Autodesk Inventor part; units mm, degrees
ref_plane "YZ Plane" through (0, 0, 0) normal (1, 0, 0) x (0, 1, 0)
ref_plane "XZ Plane" through (0, 0, 0) normal (0, 1, 0) x (-1, 0, 0)
ref_plane "XY Plane" through (0, 0, 0) normal (0, 0, 1) x (1, 0, 0)
sketch "Sketch1" plane through (0, 0, 0) normal (0, 0, 1) x (1, 0, 0)
  line L0 (-3.43, -6.35) -> (3.43, -6.35)
  line L1 (3.43, -6.35) -> (3.43, 6.35)
  line L2 (3.43, 6.35) -> (-3.43, 6.35)
  line L3 (-3.43, 6.35) -> (-3.43, -6.35)
  line L4 (-3.43, -6.35) -> (3.43, 6.35) construction
  line L5 (3.43, -6.35) -> (-3.43, 6.35) construction
  point P0 (0, 0)
  dimension "d0" = 6.86
  dimension "d1" = 12.7
extrude "Extrusion1" add sketch "Sketch1" against normal blind 8.89
sketch "Sketch2" plane through (0, 0, 0) normal (0, 0, 1) x (1, 0, 0)
  circle A0 centre (0, 0) radius 3.175
  dimension "d35" = 6.35
extrude "Extrusion2" add sketch "Sketch2" along normal blind 8.89
sketch "Sketch3" plane through (0, 0, -8.89) normal (0, 0, -1) x (-1, 0, 0)
  line L0 (-1.015, -0.38) -> (1.015, -0.38)
  line L1 (1.015, -0.38) -> (1.015, 0.38)
  line L2 (1.015, 0.38) -> (-1.015, 0.38)
  line L3 (-1.015, 0.38) -> (-1.015, -0.38)
  line L4 (-1.015, -0.38) -> (1.015, 0.38) construction
  line L5 (1.015, -0.38) -> (-1.015, 0.38) construction
  line L6 (-1.015, -5.08) -> (1.015, -5.08)
  line L7 (1.015, -5.08) -> (1.015, -4.32)
  line L8 (1.015, -4.32) -> (-1.015, -4.32)
  line L9 (-1.015, -4.32) -> (-1.015, -5.08)
  line L10 (-1.015, -5.08) -> (1.015, -4.32) construction
  line L11 (1.015, -5.08) -> (-1.015, -4.32) construction
  line L12 (-1.015, -9.78) -> (1.015, -9.78) construction
  line L13 (1.015, -9.78) -> (1.015, -9.02) construction
  line L14 (1.015, -9.02) -> (-1.015, -9.02) construction
  line L15 (-1.015, -9.02) -> (-1.015, -9.78) construction
  line L16 (-1.015, -9.78) -> (1.015, -9.02) construction
  line L17 (1.015, -9.78) -> (-1.015, -9.02) construction
  line L18 (-1.015, 4.32) -> (1.015, 4.32)
  line L19 (1.015, 4.32) -> (1.015, 5.08)
  line L20 (1.015, 5.08) -> (-1.015, 5.08)
  line L21 (-1.015, 5.08) -> (-1.015, 4.32)
  line L22 (-1.015, 4.32) -> (1.015, 5.08) construction
  line L23 (1.015, 4.32) -> (-1.015, 5.08) construction
  point P0 (0, 0)
  point P1 (0, 4.7)
  dimension "d6" = 2.03
  dimension "d7" = 0.76
  dimension "d10" = 4.7
  dimension "d17" = 4.7
extrude "Extrusion3" add sketch "Sketch3" along normal blind 3.96
sketch "Sketch4" plane through (-1.015, 5.08, -8.89) normal (0, 1, 0) x (1, 0, 0)
  line L0 (2.03, 0) -> (2.03, 3.96)
  line L1 (0, 3.96) -> (2.03, 3.96)
  circle A0 centre (1.015, 2.96) radius 0.5
  point P0 (1.015, -8.89)
  dimension "d24" = 1
  dimension "d25" = 1
  dimension "d26" = 1.015
extrude "Extrusion4" cut sketch "Sketch4" against normal through all
sketch "Sketch6" plane through (0, 0, 8.89) normal (0, 0, 1) x (1, 0, 0)
  circle A0 centre (0, 0) radius 1.46
  circle A1 centre (0, 0) radius 3.175
  dimension "d29" = 2.92
extrude "Extrusion5" add sketch "Sketch6" along normal blind 10.41 contours A0
fillet "Fillet1" radius 1.46 1 edges at (-1.46, 0, 19.3)
thread "Thread1"
sketch "Sketch7" plane through (-1.015, -5.08, -8.89) normal (0, -1, 0) x (1, 0, 0)
  circle A0 centre (1.015, -2.96) radius 0.5
sketch "Sketch8" plane through (-1.015, -0.38, -8.89) normal (0, -1, 0) x (1, 0, 0)
  circle A0 centre (1.015, -2.96) radius 0.5
sketch "Sketch9" plane through (-1.015, 4.32, -8.89) normal (0, -1, 0) x (1, 0, 0)
  circle A0 centre (1.015, -2.96) radius 0.5
properties part number "1MS2" material "Aluminum"
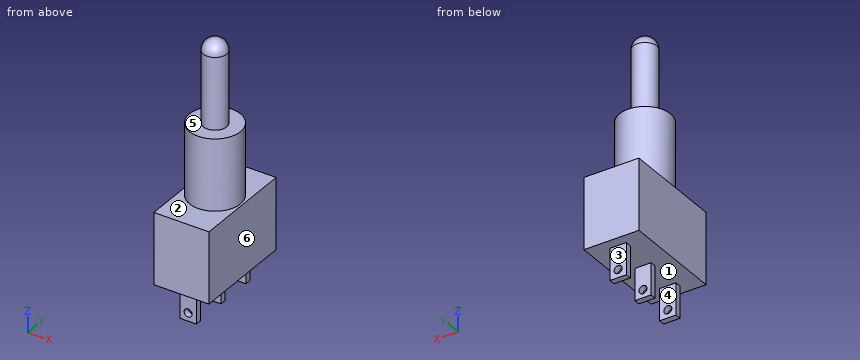
The listing builds one solid part. Answer for the finished solid, in the listing's coordinates (mm). Face numbers are marked on the shaded views. A direction names the side the tool comes from. Give positions to 0.01 mm unless a question says otherwise; leave off trailing zeros. Write each loop counter-clockwise with the first axis right and the second up, starting at its lowest first coordinate (ties: lowest second). Pieces come first, ordered by that corner, then holes. Notation, with made-up numbers: (-13.5, -2.75) - (40.5, -2.75) arc R13 cw to (40.5, 20.25) - close; hole circle Ø1 at (-28, 25.5). An arc over 180 degrees is marked (long way). Use a Markdown table: item, result.
1. A tool of negligible diameter and unlimited length cuts with its end or side. For the marked faces 4, 5 and 6, from which of +Z, -Z, +X, -X, +Y, -Y can it reach the whole face along a straight path? Write none if from no direction.
Values follow:
| item | result |
|---|---|
| face 4 | -Z, +X, -X |
| face 5 | +Z |
| face 6 | +Z, -Z, +X, +Y, -Y |
2. Each of these flat-tipped pins is pushed along its axis until it touches: P1, Ø2, axis at x = 0.5, z = -11, coming from the +Y side; P2, Ø2, axis at x = 0.5, z = -10, coming from the -Y side; P3, Ø0.8, axis at y = -4.5, z = -10.5, coming from the +X side (3 decimals). Where does it stop, or does it pass through?
Values follow:
| item | result |
|---|---|
| P1 | stops at y = 5.08 |
| P2 | stops at y = -5.08 |
| P3 | stops at x = 1.015 |
3. Section B-B on y = 0 is taken. Write down the section's boundary in (x, z) (3 decimals), plus the area to 3 significant figures.
Values follow:
| item | result |
|---|---|
| outline | (-3.43, -8.89) - (-1.015, -8.89) - (-1.015, -12.85) - (1.015, -12.85) - (1.015, -8.89) - (3.43, -8.89) - (3.43, 0) - (3.175, 0) - (3.175, 8.89) - (1.46, 8.89) - (1.46, 17.84) arc R1.46 ccw to (-1.46, 17.84) - (-1.46, 8.89) - (-3.175, 8.89) - (-3.175, 0) - (-3.43, 0) - close; hole circle Ø1 at (0, -11.85) |
| area | 154 mm² |
4. Section C-C on x = -2 is taken. Write down the section's boundary in (y, z), plus the area to 3 significant figures.
Values follow:
| item | result |
|---|---|
| outline | (-6.35, -8.89) - (6.35, -8.89) - (6.35, 0) - (2.47, 0) - (2.47, 8.89) - (-2.47, 8.89) - (-2.47, 0) - (-6.35, 0) - close |
| area | 157 mm² |
5. Section D-D on x = 0 is taken. Count the separate pieces of the cut face and the enclosed holes in it, plus the area to 3 significant figures.
Values follow:
| item | result |
|---|---|
| separate pieces | 4 |
| enclosed holes | 0 |
| area | 206 mm² |
6. Section A-A on z = -11.85 is taken. Write down the section's boundary in (x, y) (3 decimals), plus the area to 3 significant figures.
Values follow:
| item | result |
|---|---|
| outline | (-1.015, -5.08) - (-0.5, -5.08) - (-0.5, -4.32) - (-1.015, -4.32) - close; (-1.015, -0.38) - (-0.5, -0.38) - (-0.5, 0.38) - (-1.015, 0.38) - close; (-1.015, 4.32) - (-0.5, 4.32) - (-0.5, 5.08) - (-1.015, 5.08) - close; (0.5, -5.08) - (1.015, -5.08) - (1.015, -4.32) - (0.5, -4.32) - close; (0.5, -0.38) - (1.015, -0.38) - (1.015, 0.38) - (0.5, 0.38) - close; (0.5, 4.32) - (1.015, 4.32) - (1.015, 5.08) - (0.5, 5.08) - close |
| area | 2.35 mm² |
7. For a pull along Y with two mould halves and no side action, classify the marked faces 1, 2 and 3 as released by +Y, released by -Y, zero draft, split by the parting line, or undercut.
Values follow:
| item | result |
|---|---|
| face 1 | undercut |
| face 2 | zero draft |
| face 3 | released by +Y |
8. Find the intervals of material crossed by probe 1 along Z at (x, y) = (0, -4.6); probe 2 along Z at (x, y) = (-2.25, 5); probe 3 along X at (y, z) = (-4.55, -11.85) (3 decimals), in increasing order. Write a range as from..to.
Values follow:
| item | result |
|---|---|
| probe 1 | z = -12.85..-12.35, -11.35..0 |
| probe 2 | z = -8.89..0 |
| probe 3 | x = -1.015..-0.5, 0.5..1.015 |
